Source: CAD feature listing. Evaluate the final solid. Frame: model axes, mm. Coordinates: 2 decimals unless noted, no trailing zeros. Order: outer loops, then holes, each group sorted by start corner. A loop starts at its lowest first (then second) coordinate and runs counter-clockwise, first axis right, second up. Notation, with made-up numbers: (34.25, 50.5) -> (41.25, 50.5) arc R16 ccw to (41.25, 55.5) -> close; hole circle Ø4 at (62, 61.5). An arc over 180 degrees is marked (long way). Put each result on its own line as item: value.
from build123d import *

# Parameters (mm, degrees)
F0_W     = 5
F0_H     = 150
F1_DEPTH = 5
F2_R     = 1.5
F3_DEPTH = 9
F5_SIZE  = 3


with BuildPart() as f1:
    # F0 (on Top) → F1 (new body)
    with BuildSketch(Plane.XY):
        Rectangle(F0_W, F0_H)
        Polygon((-2.5, 75), (2.5, 75), (7.5, 75), (7.5, 88.5), (4.5, 88.5), (4.5, 78.5), (0, 78.5), (-4.5, 78.5), (-4.5, 88.5), (-7.5, 88.5), (-7.5, 75), align=None)
    extrude(amount=F1_DEPTH)

    # F2 (on face) → F3 (join, through all)
    with BuildSketch(Plane(origin=(4.5, 0, 0), x_dir=(0, -1, 0), z_dir=(-1, 0, 0))):
        with Locations((-85.8986780643, 2.5)):
            Circle(F2_R)
    extrude(amount=F3_DEPTH)

    # F4: F1 across plane


with BuildPart() as f1_1:
    add(f1.part)
    add(f1.part.mirror(Plane.XZ))

    # F5
    f5_edges = [f1_1.edges().sort_by_distance(p)[0] for p in [
        (-7.5, 75, 2.5),
        (7.5, 75, 2.5),
        (-7.5, -75, 2.5),
        (7.5, -75, 2.5),
    ]]
    chamfer(f5_edges, length=F5_SIZE)


solid = f1_1.part
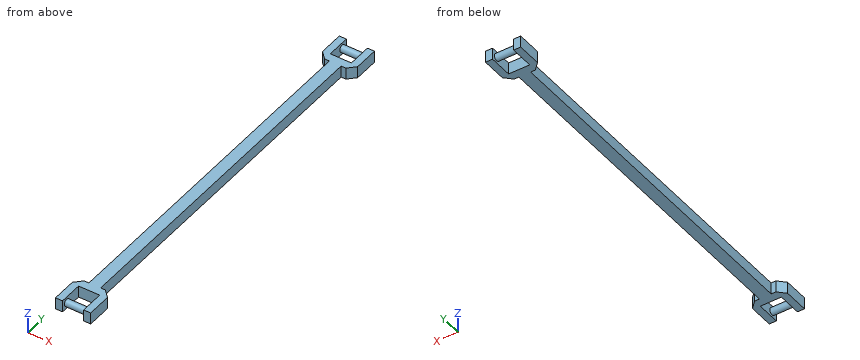
1. Ray query, line 1 along Y through (x, z) = (-4, 0.4); line 2 along Y through (x, z) = (3.5, 1.4); line 3 along Y through (x, z) = (2, 4.75). Return the intervals inside material, ascending.
Numbers:
line 1: y = -78.5 to -75, 75 to 78.5
line 2: y = -86.92 to -84.88, -78.5 to -75, 75 to 78.5, 84.88 to 86.92
line 3: y = -78.5 to 78.5
2. First-contact query: pin 1 (0.6 mm diameter, centred on x = 4, z = 2, fed in from +Y); pin 2 (2.5 mm diameter, centred on y = 14.5, z = 1.5, fed in from -X); pin 3 (1.5 mm diameter, centred on x = -2, z = 3.5, fed in from -Y). Flat tips, straight axial feed; report the tip coordinate or a pass-through.
Numbers:
pin 1: stops at y = 87.39
pin 2: stops at x = -2.5
pin 3: stops at y = -87.38
3. Cut plane B-B on y = -61. Output: boundary loops of the cut face in (x, z), plus the area to 3 significant figures.
Numbers:
outline: (-2.5, 0) -> (2.5, 0) -> (2.5, 5) -> (-2.5, 5) -> close
area: 25.0 mm2
4. Cut plane A-A on z = 2.5. Count the separate pieces of the cut face and the enclosed holes in it, plus the area to 3 significant figures.
Numbers:
separate pieces: 1
enclosed holes: 2
area: 1,010 mm2
